The model under review builds one solid part; all positions refer to its coordinate system, in mm. A direction names the side the tool comes from. Round coordinates to 2 decimals unless told otherwise and drop trailing zeros. Write each loop counter-clockwise with the first axis right and the second up, starting at its lowest first coordinate (ties: lowest second). Pieces come first, ordered by that corner, then holes. Notation, with made-up numbers: (70.25, 19.5) - (85.25, 19.5) arc R15 ccw to (85.25, 25.5) - close; hole circle Ø4 at (44, 0.5). An arc over 180 degrees is marked (long way). Return JSON: item names as keys, results as strings.
Autodesk Inventor part; units mm, degrees
ref_plane "YZ Plane" through (0, 0, 0) normal (1, 0, 0) x (0, 1, 0)
ref_plane "XZ Plane" through (0, 0, 0) normal (0, 1, 0) x (-1, 0, 0)
ref_plane "XY Plane" through (0, 0, 0) normal (0, 0, 1) x (1, 0, 0)
sketch "Sketch1" plane through (0, 0, 0) normal (0, 0, 1) x (1, 0, 0)
  arc A0 (-14, 0) -> (14, 0) centre (0, 0) ccw
  line L0 (-14, 0) -> (-14, 90)
  line L1 (-14, 90) -> (-22, 90)
  line L2 (-22, 90) -> (-22, 0)
  arc A1 (-22, 0) -> (22, 0) centre (0, 0) ccw
  line L3 (0, 0) -> (0, -14)
  line L4 (14, 0) -> (14, 90)
  line L5 (14, 90) -> (22, 90)
  line L6 (22, 90) -> (22, 0)
  dimension "d0" = 14
  dimension "d1" = 90
  dimension "d2" = 8
extrude "Extrusion1" add sketch "Sketch1" along normal mid plane 45
hole "Hole1" at (22, 70, 0) direction (-1, 0, 0) diameter 21 end through all
fillet "Fillet1" radius 20 4 edges at (18, 90, 22.5) (18, 90, -22.5) (-18, 90, -22.5) (-18, 90, 22.5)
properties part number "Suspension_Clamp_U-Clevis"
(1) Add section B-B (y = -9.5). Write out the cut boundary in (x, z).
Filled in:
{"outline": "(-19.84, -22.5) - (-10.28, -22.5) - (-10.28, 22.5) - (-19.84, 22.5) - close; (10.28, -22.5) - (19.84, -22.5) - (19.84, 22.5) - (10.28, 22.5) - close"}
(2) Add section C-C (x = -19). Write out the cut boundary in (y, z), plus the area to 3 significant figures.
Filled in:
{"outline": "(-11.09, -22.5) - (70, -22.5) arc R20 ccw to (90, -2.5) - (90, 2.5) arc R20 ccw to (70, 22.5) - (-11.09, 22.5) - close; hole circle Ø21 at (70, 0)", "area": "4,030 mm2"}
(3) Add section D-D (z = 18.5). Write out the cut boundary in (x, y).
Filled in:
{"outline": "(-22, 0) arc R22 ccw to (22, 0) - (22, 82) - (14, 82) - (14, 0) arc R14 cw to (-14, 0) - (-14, 82) - (-22, 82) - close"}
(4) Add section A-A (z = 0). Write out the cut boundary in (x, y).
Filled in:
{"outline": "(-22, 0) arc R22 ccw to (22, 0) - (22, 59.5) - (14, 59.5) - (14, 0) arc R14 cw to (-14, 0) - (-14, 59.5) - (-22, 59.5) - close; (-22, 80.5) - (-14, 80.5) - (-14, 90) - (-22, 90) - close; (14, 80.5) - (22, 80.5) - (22, 90) - (14, 90) - close"}
(5) Mouldability with a two-part tool opening along Z and no side actions: class faces 3 (the cylindrical face through (-18.056, 61.146, -5.645)), 4 (the cylindrical face through (0, -14, 0)), 5 (the flat face through (14.4, 24.6, -22.5)) as released by +Z, released by -Z, zero draft, split by the parting line, or undercut.
Filled in:
{"face 3": "undercut", "face 4": "zero draft", "face 5": "released by -Z"}
(6) Clearance check with flat-ended pins moving along their axes: pin 1 Ø3 at (y, z) = (-6, 16.5) entering from -X; pin 2 Ø12 at (x, z) = (-3.5, 0.5) entering from +Y; pin 3 Ø5 at (x, z) = (3.5, -13) entering from -Y. State where each tip first meets the part, or that it passes through.
Filled in:
{"pin 1": "stops at x = -21.53", "pin 2": "stops at y = -10.28", "pin 3": "stops at y = -21.98"}
(7) For faces 1 (the flat face through (14, 44, 0)), 2 (the flat face through (-18, 90, 0)), list the 3-axis set-ups (+Z, -Z, +X, -X, +Y, -Y) from which the entire face can be reached by the end or side of a thin tool; tool diameter is ignored.
Filled in:
{"face 1": "+Z, -Z, +Y", "face 2": "+Z, -Z, +X, -X, +Y"}
(8) Wall thickness on line 1 (X direction, y = 9.5, z = 7.5); line 2 (Z direction, x = 17.25, y = 70); line 3 (X direction, y = -9.5, z = 8): over which ranges is each line inside the solid? List them lowest first.
Filled in:
{"line 1": "x = -22 to -14, 14 to 22", "line 2": "z = -22.5 to -10.5, 10.5 to 22.5", "line 3": "x = -19.84 to -10.28, 10.28 to 19.84"}
